```python
from build123d import *

# Parameters (mm, degrees)
SKETCH1_R           = 3
SKETCH1_R_2         = 1.7
BOSS_EXTRUDE1_DEPTH = 40
FILLET1_R           = 10
SKETCH2_W           = 2.6
SKETCH2_H           = 5
CUT_EXTRUDE1_DEPTH  = 7
SKETCH3_W           = 2.6
SKETCH3_H           = 5
CUT_EXTRUDE2_DEPTH  = 11


with BuildPart() as part:
    # Sketch1 → Boss-Extrude1 (new body)
    with BuildSketch(Plane.ZY.offset(-20)):
        Polygon((2, 17), (-27.5, 17), (-27.5, 127), (-22.5, 127), (-22.5, 39), (2, 39), align=None)
        with Locations(Location((-11.25, 24, 0), (0, 0, 90))):
            Circle(SKETCH1_R, mode=Mode.SUBTRACT)
        with Locations(Location((-2.5, 31, 0), (0, 0, 90))):
            Circle(SKETCH1_R_2, mode=Mode.SUBTRACT)
        with Locations(Location((-20, 31, 0), (0, 0, 90))):
            Circle(SKETCH1_R_2, mode=Mode.SUBTRACT)
    extrude(amount=BOSS_EXTRUDE1_DEPTH)

    # Fillet1
    fillet1_edges = [part.edges().sort_by_distance(p)[0] for p in [
        (0, 39, -22.5),
    ]]
    fillet(fillet1_edges, radius=FILLET1_R)

    # Sketch2 → Cut-Extrude1 (cut)
    with BuildSketch(Plane.XY.offset(2)):
        with Locations((15.7, 31)):
            Rectangle(SKETCH2_W, SKETCH2_H)
        with Locations((-15.7, 31)):
            Rectangle(SKETCH2_W, SKETCH2_H)
    extrude(amount=-CUT_EXTRUDE1_DEPTH, mode=Mode.SUBTRACT)

    # Sketch3 → Cut-Extrude2 (cut)
    with BuildSketch(Plane(origin=(0, 0, -27.5), x_dir=(-1, 0, 0), z_dir=(0, 0, -1))):
        with Locations((15.7, 31)):
            Rectangle(SKETCH3_W, SKETCH3_H)
        with Locations((-15.7, 31)):
            Rectangle(SKETCH3_W, SKETCH3_H)
    extrude(amount=-CUT_EXTRUDE2_DEPTH, mode=Mode.SUBTRACT)


solid = part.part
```
Read the model definition and answer for the solid it produces. Units are mm, in the model's axes. A direction names the side the tool comes from. Round coordinates to 2 decimals unless told otherwise and drop trailing zeros. Write each loop counter-clockwise with the first axis right and the second up, starting at its lowest first coordinate (ties: lowest second). Pieces come first, ordered by that corner, then holes. Notation, with made-up numbers: M 89,40 L 103,40 A24 ccw 103,59 Z; hole C 1.25,16.5 d11. An arc over 180 degrees is marked long. One line per item, written item: value.
Q1. For a pull along Y with two mould halves and no side action, classify faces 1 (the flat face through (-16, 31, -16.5)), 2 (the flat face through (0, 17, -13)), 3 (the flat face through (0, 71, -27.5)) as +Y half, -Y half, draft (parallel to the pull), parting line (faces both ways), or undercut.
Data:
face 1: undercut
face 2: -Y half
face 3: draft
Q2. Find section B-B on x = 3. Write down the section's boundary in (y, z).
Data:
outline: M 17,-27.5 L 127,-27.5 L 127,-22.5 L 49,-22.5 A10 cw 39,-12.5 L 39,2 L 17,2 Z; hole C 24,-11.25 d6; hole C 31,-20 d3.4; hole C 31,-2.5 d3.4
Q3. Straight lines are drawn through the part: line 1 (Z direction, x = 19.05, y = 31); line 2 (X direction, y = 29.5, z = -25.25); line 3 (Y direction, x = -1, z = -13.5). For each, find the intervals that lie inside material, in ascending order. Write a range as [from, to].
Data:
line 1: [-27.5, -21.7], [-18.3, -4.2], [-0.8, 2]
line 2: [-20, -17], [-14.4, 14.4], [17, 20]
line 3: [17, 22.02], [25.98, 39.05]
Q4. Find section C-C on z = -11.25. Write down the section's boundary in (x, y).
Data:
outline: M -20,17 L 20,17 L 20,21 L -20,21 Z; M -20,27 L 20,27 L 20,39 L -20,39 Z
Q5. Find section A-A on y = 24. Write down the section's boundary in (x, z), plus the area to 3 significant figures.
Data:
outline: M -20,-27.5 L 20,-27.5 L 20,-14.25 L -20,-14.25 Z; M -20,-8.25 L 20,-8.25 L 20,2 L -20,2 Z
area: 940 mm2
Q6. Flat-ended cylindrical pins translate along their axes: pin 1 Ø10 at (x, y) = (-9.5, 58) entering from +Z; pin 2 Ø1 at (x, z) = (-1.5, -2.5) entering from +Y; pin 3 Ø0.8 at (x, y) = (-16, 32) entering from +Z; pin 4 Ø4.5 at (y, z) = (31, -20) entering from +X. Find the tip coordinate at first contact, or state that the pin passes through.
Data:
pin 1: z = -22.5
pin 2: y = 39
pin 3: z = -5
pin 4: x = 20
Q7. Find section D-D on z = 0.25. Write down the section's boundary in (x, y).
Data:
outline: M -20,17 L 20,17 L 20,39 L -20,39 Z; hole M -17,28.5 L -14.4,28.5 L -14.4,33.5 L -17,33.5 Z; hole M 14.4,28.5 L 17,28.5 L 17,33.5 L 14.4,33.5 Z
Q8. Which of the six approach directions +Z, -Z, +X, -X, +Y, -Y give full straight-line access (tool end or side, diameter ignored) to faces 4 (the cylindrical face through (0.2, 32.62, -3.01)), 5 (the flat face through (-16, 28.5, -1)), 6 (the flat face through (17, 31, -22))?
Data:
face 4: +X, -X
face 5: +Z
face 6: -Z
